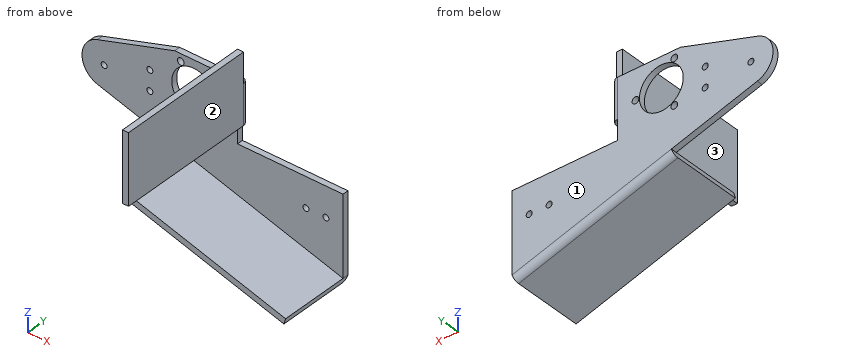
from build123d import *

# Parameters (mm, degrees)
ESQUISSE3_R        = 1.5
ESQUISSE3_R_2      = 11
ESQUISSE3_R_3      = 1.7
BOSS_EXTRU_3_DEPTH = 3
ESQUISSE6_W        = 3
ESQUISSE6_H        = 35
BOSS_EXTRU_4_DEPTH = 70
BOSS_EXTRU_5_DEPTH = 35
CONG_1_R           = 3


with BuildPart() as part:
    # Esquisse3 → Boss.-Extru.3 (new body)
    with BuildSketch(Plane.XZ):
        with BuildLine():
            Line((-464.844143116, -40.359876935), (-411.844143116, -40.359876935))
            Line((-411.844143116, -40.359876935), (-411.844143116, -80.359876935))
            Line((-411.844143116, -80.359876935), (-412.696301805, -83.236302767))
            Line((-412.696301805, -83.236302767), (-492.696301805, -59.535815029))
            Line((-492.696301805, -59.535815029), (-491.844143116, -56.659389197))
            Line((-491.844143116, -56.659389197), (-534.975651854, -43.881416773))
            ThreePointArc((-534.975651854, -43.881416773), (-542.943725497, -33.306292776), (-535.160059098, -22.594711075))
            Line((-535.160059098, -22.594711075), (-496.344143116, -10.359876935))
            Line((-496.344143116, -10.359876935), (-461.844143116, -10.359876935))
            Line((-461.844143116, -10.359876935), (-461.844143116, -30.359876935))
            Line((-461.844143116, -30.359876935), (-464.844143116, -30.359876935))
            Line((-464.844143116, -30.359876935), (-464.844143116, -40.359876935))
        make_face()
        with Locations((-531.814143116, -33.209876935)):
            Circle(ESQUISSE3_R, mode=Mode.SUBTRACT)
        with Locations((-508.844143116, -35.113476935)):
            Circle(ESQUISSE3_R, mode=Mode.SUBTRACT)
        with Locations((-508.844143116, -25.113476935)):
            Circle(ESQUISSE3_R, mode=Mode.SUBTRACT)
        with Locations((-486.844143116, -25.359876935)):
            Circle(ESQUISSE3_R_2, mode=Mode.SUBTRACT)
        with Locations((-473.844143116, -25.359876935)):
            Circle(ESQUISSE3_R_3, mode=Mode.SUBTRACT)
        with Locations((-493.344143116, -36.618207185)):
            Circle(ESQUISSE3_R_3, mode=Mode.SUBTRACT)
        with Locations((-493.344143116, -14.101546686)):
            Circle(ESQUISSE3_R_3, mode=Mode.SUBTRACT)
        with Locations((-420.455543116, -55.359876935)):
            Circle(ESQUISSE3_R, mode=Mode.SUBTRACT)
        with Locations((-430.455543116, -55.359876935)):
            Circle(ESQUISSE3_R, mode=Mode.SUBTRACT)
    extrude(amount=BOSS_EXTRU_3_DEPTH)

    # Esquisse6 → Boss.-Extru.4 (add)
    with BuildSketch(Plane.XZ.offset(3)):
        with Locations((-463.344143116, -12.859876935)):
            Rectangle(ESQUISSE6_W, ESQUISSE6_H)
    extrude(amount=BOSS_EXTRU_4_DEPTH)

    # Esquisse9 → Boss.-Extru.5 (add)
    with BuildSketch(Plane.XZ.offset(3)):
        Polygon((-492.696301805, -59.535815029), (-412.696301805, -83.236302767), (-411.844143116, -80.359876935), (-491.844143116, -56.659389197), align=None)
    extrude(amount=BOSS_EXTRU_5_DEPTH)

    # Congé1
    cong_1_edges = [part.edges().sort_by_distance(p)[0] for p in [
        (-452.696301805, 0, -71.386058898),
        (-461.844143116, 0, -20.359876935),
    ]]
    fillet(cong_1_edges, radius=CONG_1_R)


solid = part.part
Work out the finished part from the listing and answer in its coordinate system (mm). Face numbers are marked on the shaded views. A direction names the side the tool comes from. Coordinates: 2 decimals unless noted, no trailing zeros. Loops run counter-clockwise (first coordinate to the right, second up) from the corner with the lowest first, then second, coordinate; pieces in that order, holes last. Notation, with made-up numbers: M 36,51 L 69,51 A9 ccw 69,62 Z; hole C 51.5,-16 d3. An arc over 180 degrees is marked long. Answer in a Markdown table with one row per item. Add a question column.
1. A tool of negligible diameter and unlimited length cuts with its end or side. For the marked faces 1, 2 and 3, from which of +Z, -Z, +X, -X, +Y, -Y can it reach the whole face along a straight path? Write none if from no direction.
2. Consider L1, parallel to Y at x = -469.5, z = -36.5; L2, parallel to X at y = -11.5, z = -12.5; L3, parallel to Z at x = -450.5, y = -13. Determine where each line is inside the solid, lowest interval first.
3. Find section D-D, the plane z = -5.5. Write down the section's boundary in (x, y), then the cut area to 3 significant figures.
4. Find section A-A, the plane y = -17. Write down the section's boundary in (x, z), then the cut area to 3 significant figures.
5. Find section B-B, the plane z = -28.5. Write down the section's boundary in (x, y).
6. Find section C-C, the plane y = -44. Write down the section's boundary in (x, z), then the cut area to 3 significant figures.
7. Flat-ended cylindrical pins translate along their axes: P1, Ø2.5, axis at x = -531.81, z = -33.21, coming from the -Y side; P2, Ø2.5, axis at x = -462.5, z = -5.5, coming from the +Y side; P3, Ø3.5, axis at y = -1, z = -33, coming from the +X side; P4, Ø5.5, axis at x = -493.34, z = -36.62, coming from the -Y side. Find the tip coordinate at first contact, or state that the pin passes through.
Reported:
| question | item | result |
|---|---|---|
| 1 | face 1 | +Z, -Z, +X, -X, +Y |
| 1 | face 2 | +Z, +X, +Y, -Y |
| 1 | face 3 | +Z, -X, -Y |
| 2 | L1 | y = -3 to 0 |
| 2 | L2 | x = -464.84 to -461.84 |
| 2 | L3 | z = -72.04 to -68.91 |
| 3 | outline | M -464.84,-73 L -461.84,-73 L -461.84,-3 L -464.84,-3 Z |
| 3 | area | 210 mm^2 |
| 4 | outline | M -492.7,-59.54 L -412.7,-83.24 L -411.84,-80.36 L -491.84,-56.66 Z; M -464.84,-30.36 L -461.84,-30.36 L -461.84,4.64 L -464.84,4.64 Z |
| 4 | area | 355 mm^2 |
| 5 | outline | M -541.9,-3 L -497.39,-3 L -497.39,0 L -541.9,0 Z; M -476.3,-3 L -464.84,-3 L -464.84,-73 L -461.84,-73 L -461.84,-3 A3 ccw -464.84,0 L -476.3,0 Z |
| 6 | outline | M -464.84,-30.36 L -461.84,-30.36 L -461.84,4.64 L -464.84,4.64 Z |
| 6 | area | 105 mm^2 |
| 7 | P1 | passes through |
| 7 | P2 | stops at y = -3 |
| 7 | P3 | stops at x = -464.84 |
| 7 | P4 | stops at y = -3 |
